The drawing under review shows one solid part. Ordinate dimensions are in mm from its lowest x, y, z. A direction names the side the tool comes from. Give positions to 0.01 mm unless a question says otherwise; leave off trailing zeros. Order: outer loops, then holes, each group sorted by start corner. A loop starts at its lowest first (then second) coordinate and runs counter-clockwise, first axis right, second up. Notation, with made-up numbers: (14.25, 33) -> (26.25, 33) arc R18 cw to (26.25, 41) -> close; hole circle Ø7 at (-19, 84.25). An arc over 180 degrees is marked (long way). Return JSON: item names as keys, results as strings. Group by question number.
1) To check wall thickness, follow line 1 along X through (y, z) = (1, 4.75); line 2 along Z through (x, y) = (36, 0.4); line 3 along Z through (x, y) = (42.5, 5.5). State the ranges of each line that lie inside material, in increasing order.
2) Add section B-B (z = 15.5). Give the boundary of the cut face in (x, y).
3) Add section A-A (x = 36). Give the boundary of the cut face in (y, z).
4) For the marked faces 1 and 2, list the 3-axis set-ups (+Z, -Z, +X, -X, +Y, -Y) from which the entire face can be reached by the end or side of a thin tool; tool diameter is ignored.
5) Add section D-D (z = 8.25). Give the boundary of the cut face in (x, y).
6) Insertion check: P1, Ø4, axis at x = 31, z = 19.5, coming from the +Y side; P2, Ø1, axis at x = 22, y = 2, coming from the -Z side; P3, Ø5, axis at x = 16.5, y = 8.5, coming from the +Z side; P4, Ø6, axis at x = 27, y = 8, coming from the -Z side. Each pin has a flat end and moves straight along its axis. Give the tip position at first contact, or say it passes through.
7) The part is to be moulded in two halves that separate along X. For the marked faces 3, 4 and 5, say which applies: released by +X, released by -X, zero draft, split by the parting line, or undercut.
8) Add section C-C (y = 5.5). Give the boundary of the cut face in (x, z), then the cut area to 3 significant figures.
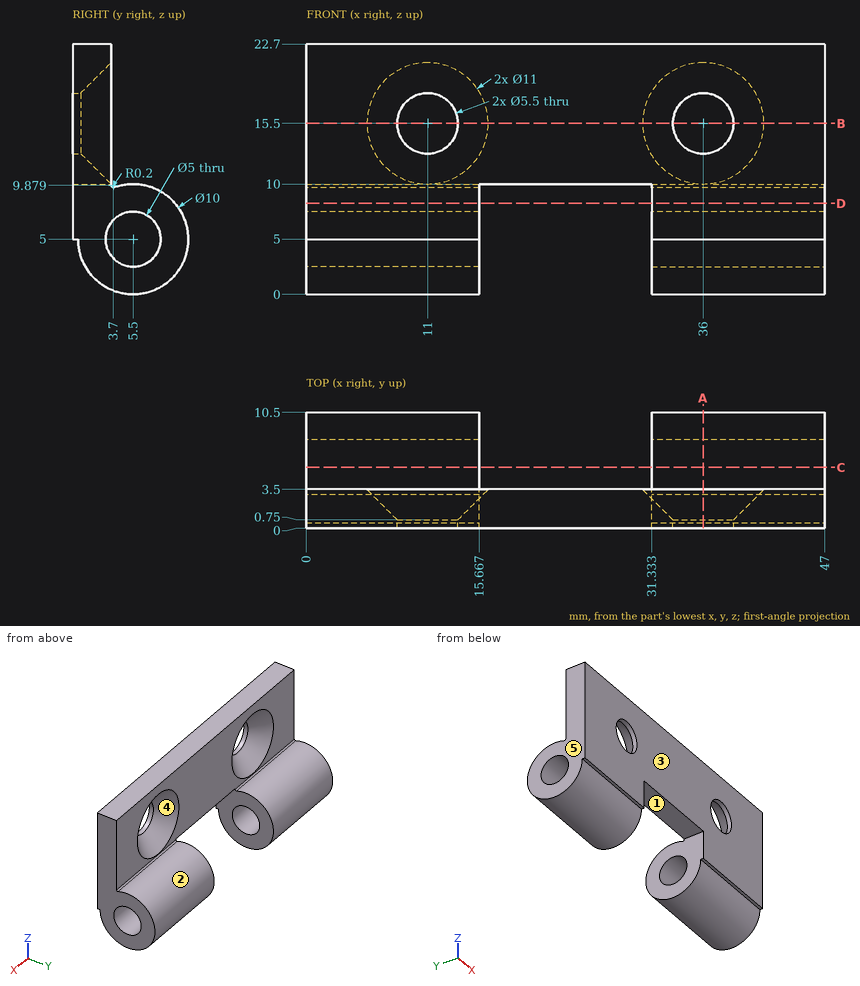
Evaluation:
{
 "1": {"line 1": "0 to 15.67, 31.33 to 47", "line 2": "5 to 12.75, 18.25 to 22.7", "line 3": "0 to 2.5, 7.5 to 10"},
 "2": {"outline": "(0, 0) -> (8.25, 0) -> (8.25, 0.75) -> (5.5, 3.5) -> (0, 3.5) -> close; (13.75, 0) -> (33.25, 0) -> (33.25, 0.75) -> (30.5, 3.5) -> (16.5, 3.5) -> (13.75, 0.75) -> close; (38.75, 0) -> (47, 0) -> (47, 3.5) -> (41.5, 3.5) -> (38.75, 0.75) -> close"},
 "3": {"outline": "(0, 5) -> (0.5, 5) arc R5 ccw (long way) to (3.77, 9.69) arc R0.2 cw to (3.5, 9.88) -> (3.5, 10) -> (0.75, 12.75) -> (0, 12.75) -> close; (0, 18.25) -> (0.75, 18.25) -> (3.5, 21) -> (3.5, 22.7) -> (0, 22.7) -> close; hole circle Ø5 at (5.5, 5)"},
 "4": {"face 1": "-Z, +Y, -Y", "face 2": "+X, -X"},
 "5": {"outline": "(0, 0) -> (15.67, 0) -> (15.67, 9.3) -> (0, 9.3) -> close; (31.33, 0) -> (47, 0) -> (47, 9.3) -> (31.33, 9.3) -> close"},
 "6": {"P1": "y = 3.5", "P2": "z = 10", "P3": "z = 9.96", "P4": "through"},
 "7": {"face 3": "zero draft", "face 4": "undercut", "face 5": "released by -X"},
 "8": {"outline": "(0, 0) -> (15.67, 0) -> (15.67, 2.5) -> (0, 2.5) -> close; (0, 7.5) -> (15.67, 7.5) -> (15.67, 10) -> (0, 10) -> close; (31.33, 0) -> (47, 0) -> (47, 2.5) -> (31.33, 2.5) -> close; (31.33, 7.5) -> (47, 7.5) -> (47, 10) -> (31.33, 10) -> close", "area": "157 mm^2"}
}
